from build123d import *

# Parameters (mm, degrees)
SKETCH1_W           = 34.925
SKETCH1_H           = 25.4
BOSS_EXTRUDE1_DEPTH = 76.2
SKETCH2_R           = 3.687507865
SKETCH2_R_2         = 4.491133618
CUT_EXTRUDE1_DEPTH  = 85.77904001


with BuildPart() as part:
    # Sketch1 → Boss-Extrude1 (new, symmetric)
    with BuildSketch(Plane(origin=(0, 0, 0), x_dir=(0, 0, -1), z_dir=(1, 0, 0))):
        Rectangle(SKETCH1_W, SKETCH1_H)
    extrude(amount=BOSS_EXTRUDE1_DEPTH, both=True)

    # Sketch2 → Cut-Extrude1 (cut, through all)
    with BuildSketch(Plane.XY.offset(17.4625)):
        with Locations((-54.290984638, 0)):
            Circle(SKETCH2_R)
        with Locations((54.290984638, 0)):
            Circle(SKETCH2_R_2)
    extrude(amount=-CUT_EXTRUDE1_DEPTH, mode=Mode.SUBTRACT)


solid = part.part
The listing builds one solid part. Answer for the finished solid, in the listing's coordinates (mm). Round coordinates to 2 decimals unless told otherwise and drop trailing zeros. Write each loop counter-clockwise with the first axis right and the second up, starting at its lowest first coordinate (ties: lowest second). Pieces come first, ordered by that corner, then holes. Notation, with made-up numbers: (62.25, 70) - (104.25, 70) arc R31 ccw to (104.25, 94) - close; hole circle Ø6 at (-17.5, 27). An arc over 180 degrees is marked (long way). Use a Markdown table: item, result. Add a question column.
1. For a pull along X with two mould halves and no side action, classify faces 1 (the face through (1, 0, 17.462)), 2 (the face through (49.804, 0.197, 0.244)), 3 (the face through (-76.2, 0, 0)) as +X half, -X half, draft (parallel to the pull), parting line (faces both ways), or undercut.
2. Consider line 1 (X direction, y = -1, z = -15); line 2 (Y direction, x = -51, z = -2); line 3 (Y direction, x = -57.5, z = 7.5). Determine where each line is inside the solid, lowest interval first.
3. A flat-ended cylindrical pin translates along its axis: P1, Ø12, axis at x = -54.29, y = 0, coming from the +Z side. Find the tip coordinate at first contact, or state that the pin passes through.
4. The part is cut by section A-A (y = 0). Write down the section's boundary in (x, z).
5. The part is cut by section C-C (z = 13). Write down the section's boundary in (x, y), and give its area (3 significant figures).
6. The part is cut by section B-B (x = -56). Write down the section's boundary in (y, z).
7. The part is cut by section D-D (x = 51.5). Write down the section's boundary in (y, z), and give its area (3 significant figures).
Reported:
| question | item | result |
|---|---|---|
| 1 | face 1 | draft |
| 1 | face 2 | undercut |
| 1 | face 3 | -X half |
| 2 | line 1 | -76.2 to -57.84, -50.74 to 49.91, 58.67 to 76.2 |
| 2 | line 2 | -12.7 to -1.66, 1.66 to 12.7 |
| 2 | line 3 | -12.7 to -1.82, 1.82 to 12.7 |
| 3 | P1 | z = 17.46 |
| 4 | outline | (-76.2, -17.46) - (-57.98, -17.46) - (-57.98, 17.46) - (-76.2, 17.46) - close; (-50.6, -17.46) - (49.8, -17.46) - (49.8, 17.46) - (-50.6, 17.46) - close; (58.78, -17.46) - (76.2, -17.46) - (76.2, 17.46) - (58.78, 17.46) - close |
| 5 | outline | (-76.2, -12.7) - (76.2, -12.7) - (76.2, 12.7) - (-76.2, 12.7) - close; hole circle Ø7.38 at (-54.29, 0); hole circle Ø8.98 at (54.29, 0) |
| 5 | area | 3,760 mm^2 |
| 6 | outline | (-12.7, -17.46) - (-3.27, -17.46) - (-3.27, 17.46) - (-12.7, 17.46) - close; (3.27, -17.46) - (12.7, -17.46) - (12.7, 17.46) - (3.27, 17.46) - close |
| 7 | outline | (-12.7, -17.46) - (-3.52, -17.46) - (-3.52, 17.46) - (-12.7, 17.46) - close; (3.52, -17.46) - (12.7, -17.46) - (12.7, 17.46) - (3.52, 17.46) - close |
| 7 | area | 641 mm^2 |
